Build history of the part. All positions in model axes, mm. A direction names the side the tool comes from. Round coordinates to 2 decimals unless told otherwise and drop trailing zeros. Write each loop counter-clockwise with the first axis right and the second up, starting at its lowest first coordinate (ties: lowest second). Pieces come first, ordered by that corner, then holes. Notation, with made-up numbers: M 15.5,-18.75 L 44.5,-18.75 A25 ccw 44.5,16.25 Z; hole C 33.25,13 d10. An arc over 180 degrees is marked long. Write item = value, one per line.
from build123d import *

# Parameters (mm, degrees)
SWEEP1_PROFILE_R         = 7.5
BOSS_EXTRUDE1_REACH      = 188.649
BOSS_EXTRUDE1_END_RADIUS = 7.5
SKETCH10_R               = 7.5
SKETCH11_R               = 7.5
SKETCH11_R_2             = 5
CUT_EXTRUDE1_DEPTH       = 15


with BuildPart() as part:
    # Sweep1: sweep along a path in Sketch1
    with BuildLine(Plane.XY) as sweep1_path:
        Line((-9.568747019, 51.5), (14.70492956, 51.5))
        ThreePointArc((14.70492956, 51.5), (20.88607003, 49.360884333), (24.422775616, 43.858700499))
        Line((24.422775616, 43.858700499), (44.568406684, -39.141299501))
        ThreePointArc((44.568406684, -39.141299501), (42.711444961, -47.68114047), (34.850560628, -51.5))
        Line((34.850560628, -51.5), (-29.714378087, -51.5))
        ThreePointArc((-29.714378087, -51.5), (-37.57526242, -47.68114047), (-39.432224142, -39.141299501))
        Line((-39.432224142, -39.141299501), (-19.286593074, 43.858700499))
        ThreePointArc((-19.286593074, 43.858700499), (-15.749887488, 49.360884333), (-9.568747019, 51.5))
    # Sweep1 profile (on start of the path) → Sweep1 (sweep)
    with BuildSketch(Plane(origin=(-9.568747019, 51.5, 0), x_dir=(0, 1, 0), z_dir=(1, 0, 0))):
        Circle(SWEEP1_PROFILE_R)
    sweep(path=sweep1_path.line)

    # Boss-Extrude1: up to this cylinder (the profile starts outside it)
    boss_extrude1_end = Plane(origin=(0, 51.5, 0), z_dir=(1, 0, 0)) * Cylinder(BOSS_EXTRUDE1_END_RADIUS, 393.298, mode=Mode.PRIVATE)
    # Sketch10 → Boss-Extrude1 (add, up to the surface)
    with BuildSketch(Plane(origin=(0, 120, 0), x_dir=(1, 0, 0), z_dir=(0, 1, 0)), mode=Mode.PRIVATE) as boss_extrude1_sk1:
        with Locations(Location((0, 0, 0), (0, 0, 270))):
            Circle(SKETCH10_R)
    boss_extrude1_tool1 = extrude(boss_extrude1_sk1.sketch, amount=-BOSS_EXTRUDE1_REACH, mode=Mode.PRIVATE) - boss_extrude1_end
    add(boss_extrude1_tool1.solids().sort_by_distance((0, 120, 0))[0])

    # Sketch11 → Cut-Extrude1 (cut)
    with BuildSketch(Plane(origin=(0, 120, 0), x_dir=(1, 0, 0), z_dir=(0, 1, 0))):
        with Locations(Location((0, 0, 0), (0, 0, 270))):
            Circle(SKETCH11_R)
        with Locations(Location((0, 0, 0), (0, 0, 270))):
            Circle(SKETCH11_R_2, mode=Mode.SUBTRACT)
    extrude(amount=-CUT_EXTRUDE1_DEPTH, mode=Mode.SUBTRACT)


solid = part.part
1. Tool access for faces 4 (the face through (2, -44, 0)), 5 (the face through (-5, 105, 2)): list every direction of +Z, -Z, +X, -X, +Y, -Y with a clear straight run to the whole face (end or side of a thin tool).
Responses:
face_4 = none
face_5 = +Y
2. Band-saw the part on A-A (x = 0). List the corners of the cut face in (y, z).
Responses:
outline = C -51.5,0 d15; M 51.5,-7.5 L 105,-7.5 L 105,-5 L 120,-5 L 120,5 L 105,5 L 105,7.5 L 51.5,7.5 A7.5 ccw Z
3. Probe probe 1 along Y at (x, z) = (-0.5, -0.75); probe 2 along Y at (x, z) = (8.5, 2); probe 3 along X at (y, z) = (-25.5, -6.25). List the from-to ranges inside material, lowest first.
Responses:
probe_1 = -58.96 to -44.04, 44.04 to 120
probe_2 = -58.73 to -44.27, 44.27 to 58.73
probe_3 = -40.39 to -31.86, 36.99 to 45.52
4. Band-saw the part on B-B (z = -2.25). List the corners of the cut face in (x, y).
Responses:
outline = M -46.38,-37.45 A17.15 ccw -29.71,-58.65 L 34.85,-58.65 A17.15 ccw 51.52,-37.45 L 31.38,45.55 A17.15 ccw 14.7,58.65 L 7.15,58.65 L 7.15,105 L 4.47,105 L 4.47,120 L -4.47,120 L -4.47,105 L -7.15,105 L -7.15,58.65 L -9.57,58.65 A17.15 ccw -26.24,45.55 Z; hole M -32.48,-40.83 A2.85 ccw -29.71,-44.35 L 34.85,-44.35 A2.85 ccw 37.62,-40.83 L 17.47,42.17 A2.85 ccw 14.7,44.35 L -9.57,44.35 A2.85 ccw -12.33,42.17 Z
5. Mould opens along X. For faces 1 (the face through (-4.88, 112.6, -1.08)), 2 (the face through (0, 120, 0)), 3 (the face through (41.59, 3.47, 2.25)) say: pulls with the +X half, pulls with the -X half, needs draft (parallel to the pull), parting line crosses it, or undercut.
Responses:
face_1 = parting line crosses it
face_2 = needs draft
face_3 = undercut
6. Band-saw the part on C-C (y = 97). List the corners of the cut face in (x, z), plus the area to 3 significant figures.
Responses:
outline = C 0,0 d15
area = 177 mm²
7. Flat gauge pins, fed straight in: pin 1 (6 mm diameter, centred on y = -12.5, z = 4, fed in from -X); pin 2 (1 mm diameter, centred on y = 50, z = -2.5, fed in from +X) (3 decimals); pin 3 (1.5 mm diameter, centred on x = 16, z = -3, fed in from -Y). Where does each tip first touch, or does it go through?
Responses:
pin_1 = -40.95
pin_2 = 29.845
pin_3 = -58.65
